```python
from build123d import *

# Parameters (mm, degrees)
F0_W      = 101.6
F0_H      = 127
F1_DEPTH  = 6.35
F2_W      = 6.35
F2_H      = 6.35
F3_DEPTH  = 6.351
F5_DEPTH  = 6.351
F6_W      = 3.175
F6_H      = 3.175
F7_DEPTH  = 6.3510001
F9_DEPTH  = 34.798
F11_DEPTH = 25.4
F13_DEPTH = 25.4


with BuildPart() as f1:
    # F0 (on Front) → F1 (new body)
    with BuildSketch(Plane.XZ):
        Rectangle(F0_W, F0_H)
    extrude(amount=F1_DEPTH)

    # F2 (on face) → F3 (cut, through all)
    with BuildSketch(Plane.XZ.offset(6.35)):
        with Locations((-47.625, 53.975)):
            Rectangle(F2_W, F2_H)
        with Locations((47.625, 53.975)):
            Rectangle(F2_W, F2_H)
        with Locations((47.625, -60.325)):
            Rectangle(F2_W, F2_H)
        with Locations((-47.625, -60.325)):
            Rectangle(F2_W, F2_H)
    extrude(amount=-F3_DEPTH, mode=Mode.SUBTRACT)

    # F4 (on face) → F5 (cut, through all)
    with BuildSketch(Plane.XZ.offset(6.35)):
        with BuildLine():
            Line((-50.8, 63.5), (-50.8, 57.15))
            add(Edge.make_bspline(
                [(-3.402e-07, 63.5), (-50.8, 63.4999999575), (-50.8, 57.15)],
                knots=[4.7123889871, 4.7123889871, 4.7123889871, 6.2831853072, 6.2831853072, 6.2831853072], degree=2, weights=[1, 0.7071067836, 1]))
            Line((-3.402e-07, 63.5), (-50.8, 63.5))
        make_face()
        with BuildLine():
            add(Edge.make_bspline(
                [(50.8, 57.15), (50.8, 63.5000000425), (-3.402e-07, 63.5)],
                knots=[3.1415926536, 3.1415926536, 3.1415926536, 4.7123889871, 4.7123889871, 4.7123889871], degree=2, weights=[1, 0.7071067788, 1]))
            Line((50.8, 57.15), (50.8, 63.5))
            Line((50.8, 63.5), (-3.402e-07, 63.5))
        make_face()
    extrude(amount=-F5_DEPTH, mode=Mode.SUBTRACT)

    # F6 (on face) → F7 (cut, through all)
    with BuildSketch(Plane.XZ.offset(6.35)):
        with Locations((-42.8625, 55.5625)):
            Rectangle(F6_W, F6_H)
        with Locations((-14.2875, 55.5625)):
            Rectangle(F6_W, F6_H)
        with Locations((14.2875, 55.5625)):
            Rectangle(F6_W, F6_H)
        with Locations((42.8625, 55.5625)):
            Rectangle(F6_W, F6_H)
        with Locations((36.5125, 24.7015)):
            Rectangle(F6_W, F6_H)
        with Locations((5.3975, 24.7015)):
            Rectangle(F6_W, F6_H)
    extrude(amount=-F7_DEPTH, mode=Mode.SUBTRACT)

    # F8 (on Front) → F9 (cut)
    with BuildSketch(Plane.XZ):
        Polygon((2.9555256112, 1.8009109067), (-43.1100860449, 18.5674223729), (-44.196, 15.5838983019), (1.8696116562, -1.1826131642), align=None)
    extrude(amount=F9_DEPTH, mode=Mode.SUBTRACT)

    # F10 (on Front) → F11 (cut)
    with BuildSketch(Plane.XZ):
        Polygon((43.1100860449, -7.7964003764), (-2.9555256112, -24.5629118425), (-1.8696116562, -27.5464359135), (44.196, -10.7799244474), align=None)
    extrude(amount=F11_DEPTH, mode=Mode.SUBTRACT)

    # F12 (on Front) → F13 (cut)
    with BuildSketch(Plane.XZ):
        Polygon((2.9555256112, -50.9267345918), (-43.1100860449, -34.1602231257), (-44.196, -37.1437471967), (1.8696116562, -53.9102586628), align=None)
    extrude(amount=F13_DEPTH, mode=Mode.SUBTRACT)


solid = f1.part
```
Work out the finished part from the listing and answer in its coordinate system (mm). A direction names the side the tool comes from. Round coordinates to 2 decimals unless told otherwise and drop trailing zeros. Loops run counter-clockwise (first coordinate to the right, second up) from the corner with the lowest first, then second, coordinate; pieces in that order, holes last. Notation, with made-up numbers: (79, 55.5) -> (89, 55.5) arc R15 cw to (89, 72.5) -> close; hole circle Ø7 at (27, 2.5). An arc over 180 degrees is marked (long way). Write each question's results on one line, items separated by ' | '. Start each with the question number.
1. Find the intervals of material crossed by probe 1 along Z at (x, y) = (37, -2.25); probe 2 along Z at (x, y) = (35, -5.5); probe 3 along Z at (x, y) = (28, -5.25), in increasing order. Write a range as from..to.
2. Section A-A (z = -46) is taken. Determine the outline of the cut face in (x, y).
3. A tool of negligible diameter and unlimited length cuts with its end or side. For faces 1 (the face through (44.45, -3, -60)), 2 (the face through (-43.645, -3.131, -35.631)), 3 (the face through (46, -3, 57.15)), from which of +Z, -Z, +X, -X, +Y, -Y can it reach the whole face along a straight path? Write none if from no direction.
4. Section B-B (y = -4.5) is taken. State how many separate pieces and enclosed holes the cut face has, plus the area to 3 significant figures.
5. Given pin 1 Ø1.6 at (y, z) = (-3.5, 55) entering from -X (3 decimals); pin 2 Ø3.5 at (x, y) = (-43.5, -2.5) entering from +Z; pin 3 Ø1 at (y, z) = (-1.5, 52) entering from +X, each flat-ended and moving along its own axis, determine where each tip first touches the part or whether it passes through.
6. For a pull along X with two mould halves and no side action, classify faces 4 (the face through (12.7, -3, 56)), 5 (the face through (-48, -3, 50.8)), 6 (the face through (41.275, -3, 56)) as +X half, -X half, draft (parallel to the pull), parting line (faces both ways), or undercut.
Evaluation:
1) probe 1: z = -63.5..-13.4, -10.02..23.11, 26.29..61.5 | probe 2: z = -63.5..-14.13, -10.75..23.11, 26.29..61.75 | probe 3: z = -63.5..-16.67, -13.3..62.45
2) outline: (-50.8, -6.35) -> (-19.86, -6.35) -> (-19.86, 0) -> (-50.8, 0) -> close; (-10.58, -6.35) -> (50.8, -6.35) -> (50.8, 0) -> (-10.58, 0) -> close
3) face 1: -Z, +X, +Y, -Y | face 2: +Y, -Y | face 3: +X, +Y, -Y
4) separate pieces: 1 | enclosed holes: 7 | area: 12,100 mm2
5) pin 1: stops at x = -41.275 | pin 2: stops at z = 60.77 | pin 3: stops at x = 44.45
6) face 4: undercut | face 5: draft | face 6: +X half
